```python
from build123d import *

# Parameters (mm, degrees)
SKETCH2_W          = 13.807149041
SKETCH2_H          = 34.00821274
SKETCH2_W_2        = 8.154557823
SKETCH2_H_2        = 39.290142239
CUT_EXTRUDE1_DEPTH = 17


with BuildPart() as part:
    # Sketch1 → Revolve1 (revolve)
    with BuildSketch(Plane.XY, mode=Mode.PRIVATE) as revolve1_sk:
        with BuildLine():
            Line((-239, 15), (-187, 15))
            Line((-187, 15), (-187, 20))
            Line((-187, 20), (187, 20))
            Line((187, 20), (187, 15))
            Line((187, 15), (267, 15))
            ThreePointArc((267, 15), (268.497797314, 7.566372975), (269, 0))
            Line((269, 0), (-241, 0))
            ThreePointArc((-241, 0), (-240.497797314, 7.566372975), (-239, 15))
        make_face()
    revolve(revolve1_sk.sketch.rotate(Axis((-241, 0, 0), (1, 0, 0)), 180), axis=Axis((-241, 0, 0), (1, 0, 0)))

    # Sketch2 → Cut-Extrude1 (cut)
    with BuildSketch(Plane.ZY.offset(187)):
        with Locations((23.903574521, 0.880321583)):
            Rectangle(SKETCH2_W, SKETCH2_H)
        with Locations((-21.077278912, -2.316635745)):
            Rectangle(SKETCH2_W_2, SKETCH2_H_2)
    extrude(amount=-CUT_EXTRUDE1_DEPTH, mode=Mode.SUBTRACT)


solid = part.part
```
Work out the finished part from the listing and answer in its coordinate system (mm). A direction names the side the tool comes from. Give positions to 0.01 mm unless a question says otherwise; leave off trailing zeros. Order: outer loops, then holes, each group sorted by start corner. A loop starts at its lowest first (then second) coordinate and runs counter-clockwise, first axis right, second up.
1. Straight lines are drawn through the part: L1, parallel to Z at x = -175.5, y = -9; L2, parallel to X at y = -0.5, z = -2.5; L3, parallel to X at y = -16.5, z = 8. For each, find the intervals that lie inside material, in ascending order.
Result sheet:
L1: z = -17 to 17
L2: x = -240.94 to 268.94
L3: x = -187 to 187
2. Section D-D, the plane x = -145.5 is taken. Determine the outline of the cut face in (y, z), and give its area (3 significant figures).
Result sheet:
outline: circle Ø40 at (0, 0)
area: 1,260 mm2
3. Section B-B, the plane z = 0 is taken. Determine the outline of the cut face in (x, y).
Result sheet:
outline: (-239, -15) - (-187, -15) - (-187, -20) - (187, -20) - (187, -15) - (267, -15) arc R57.25 ccw to (267, 15) - (187, 15) - (187, 20) - (-187, 20) - (-187, 15) - (-239, 15) arc R57.25 ccw to start
4. Each of these flat-tipped pins is pushed along its axis until it touches: P1, Ø13.5, axis at x = -179.5, y = 2.5, coming from the +Z side; P2, Ø1.5, axis at y = -14, z = 9.5, coming from the -X side; P3, Ø2, axis at x = 60.5, y = 5, coming from the -Z side. Where does it stop, or does it pass through?
Result sheet:
P1: stops at z = 17
P2: stops at x = -187
P3: stops at z = -19.6
5. Section C-C, the plane x = -200.5 is taken. Determine the outline of the cut face in (y, z), and give its area (3 significant figures).
Result sheet:
outline: circle Ø30 at (0, 0)
area: 707 mm2
6. For faces 1 (the flat face through (-179, 0, 17)), 2 (the flat face through (-187, -3, 15)), 3 (the cylindrical face through (2.62, 19.98, -0.88)), 4 (the flat face through (187, -3, -15)), 5 (the flat face through (-179, 0, -17)), determine the directions among +Z, -Z, +X, -X, +Y, -Y from which every point of the face is accessible in a straight line to the end or side of a thin tool.
Result sheet:
face 1: +Z, -X, +Y, -Y
face 2: -X
face 3: +X, -X
face 4: +X
face 5: -Z, -X, +Y, -Y
7. Section A-A, the plane y = 0 is taken. Determine the outline of the cut face in (x, z).
Result sheet:
outline: (-239, -15) - (-187, -15) - (-187, -17) - (-170, -17) - (-170, -20) - (187, -20) - (187, -15) - (267, -15) arc R57.25 ccw to (267, 15) - (187, 15) - (187, 20) - (-170, 20) - (-170, 17) - (-187, 17) - (-187, 15) - (-239, 15) arc R57.25 ccw to start
